from build123d import *

# Parameters (mm, degrees)
F0_W     = 58.42
F0_H     = 31.75
F2_DEPTH = 25.4
F3_R     = 6.35
F4_T     = -3.175
F5_R     = 2.54
F6_DEPTH = 6.35
F7_R     = 1.27
F8_DEPTH = 3.81


with BuildPart() as f2:
    # F0 (on Front) → F2 (new body)
    with BuildSketch(Plane.XZ):
        Rectangle(F0_W, F0_H)
    extrude(amount=F2_DEPTH)

    # F3
    f3_edges = [f2.edges().sort_by_distance(p)[0] for p in [
        (29.21, -12.7, 15.875),
        (29.21, -12.7, -15.875),
        (-29.21, -12.7, 15.875),
        (-29.21, -12.7, -15.875),
    ]]
    fillet(f3_edges, radius=F3_R)

    # F4
    f4_openings = [f2.faces().sort_by_distance(p)[0] for p in [
        (0, -25.4, 0),
    ]]
    offset(amount=F4_T, openings=f4_openings)

    # F5 (on face) → F6 (join)
    with BuildSketch(Plane.XZ.offset(3.175)):
        with Locations((-22.86, 8.89)):
            Circle(F5_R)
        with Locations((22.86, 8.89)):
            Circle(F5_R)
        with Locations((-22.86, -8.89)):
            Circle(F5_R)
        with Locations((22.86, -8.89)):
            Circle(F5_R)
    extrude(amount=F6_DEPTH)

    # F7 (on face) → F8 (join)
    with BuildSketch(Plane.XZ.offset(9.525)):
        with Locations((-22.86, 8.89)):
            Circle(F7_R)
        with Locations((-22.86, -8.89)):
            Circle(F7_R)
        with Locations((22.86, -8.89)):
            Circle(F7_R)
        with Locations((22.86, 8.89)):
            Circle(F7_R)
    extrude(amount=F8_DEPTH)


solid = f2.part
The model under review builds one solid part; all positions refer to its coordinate system, in mm. A direction names the side the tool comes from. Give positions to 0.01 mm unless a question says otherwise; leave off trailing zeros. Write each loop counter-clockwise with the first axis right and the second up, starting at its lowest first coordinate (ties: lowest second). Pieces come first, ordered by that corner, then holes.
1. Draft analysis for pull direction X (two halves, no side actions). For faces 1 (the cylindrical face through (25.13, -14.443, 11.745)), 2 (the cylindrical face through (27.399, -12.878, 13.965)), 3 (the flat face through (0, -13, -15.875)), 4 (the flat face through (-29.21, -13, 0)), state which applies: +X half, -X half, draft (parallel to the pull), parting line (faces both ways), or undercut.
2. For P1, Ø1.3, axis at x = 23, z = 8.5, coming from the -Y side (3 decimals); P2, Ø12.5, axis at x = -8, z = 6, coming from the -Y side (3 decimals), all flat-tipped, find the tip position at first contact; note any pin that passes through.
3. Add section A-A, the plane y = -7.25. Write out the cut boundary in (x, z) (3 decimals), plus the area to 3 significant figures.
4. Add section D-D, the plane x = 17. Write out the cut boundary in (y, z) (3 decimals), plus the area to 3 significant figures.
5. Wall thickness on L1, parallel to Z at x = 10, y = -12.5 (3 decimals); L2, parallel to X at y = -9.5, z = -1 (3 decimals); L3, parallel to X at y = -5, z = 11: over which ranges is each line inside the solid? List them lowest first.
6. Add section B-B, the plane z = -3.5. Write out the cut boundary in (x, y) (3 decimals).
7. Tool access review of faces 5 (the flat face through (23, -13.335, 9)), 6 (the flat face through (0, -13, 15.875)): name each direction out of +Z, -Z, +X, -X, +Y, -Y from which nothing blocks a thin tool from reaching the whole face with its end or side.
8. Add section C-C, the plane y = -17. Write out the cut boundary in (x, z) (3 decimals).
Worked answers:
1. face 1: undercut
1. face 2: +X half
1. face 3: draft
1. face 4: -X half
2. P1: stops at y = -13.335
2. P2: stops at y = -3.175
3. outline: (-29.21, -9.525) arc R6.35 ccw to (-22.86, -15.875) - (22.86, -15.875) arc R6.35 ccw to (29.21, -9.525) - (29.21, 9.525) arc R6.35 ccw to (22.86, 15.875) - (-22.86, 15.875) arc R6.35 ccw to (-29.21, 9.525) - close; circle Ø5.08 at (-22.86, -8.89); circle Ø5.08 at (-22.86, 8.89); circle Ø5.08 at (22.86, -8.89); circle Ø5.08 at (22.86, 8.89); hole (-26.035, -9.525) arc R3.175 ccw to (-22.86, -12.7) - (22.86, -12.7) arc R3.175 ccw to (26.035, -9.525) - (26.035, 9.525) arc R3.175 ccw to (22.86, 12.7) - (-22.86, 12.7) arc R3.175 ccw to (-26.035, 9.525) - close
3. area: 587 mm2
4. outline: (-25.4, -15.875) - (0, -15.875) - (0, 15.875) - (-25.4, 15.875) - (-25.4, 12.7) - (-3.175, 12.7) - (-3.175, -12.7) - (-25.4, -12.7) - close
4. area: 242 mm2
5. L1: z = -15.875 to -12.7, 12.7 to 15.875
5. L2: x = -29.21 to -26.035, 26.035 to 29.21
5. L3: x = -29.04 to -25.67, -24.27 to -21.45, 21.45 to 24.27, 25.67 to 29.04
6. outline: (-29.21, -25.4) - (-26.035, -25.4) - (-26.035, -3.175) - (26.035, -3.175) - (26.035, -25.4) - (29.21, -25.4) - (29.21, 0) - (-29.21, 0) - close
7. face 5: -Y
7. face 6: +Z, +X, -X, +Y, -Y
8. outline: (-29.21, -9.525) arc R6.35 ccw to (-22.86, -15.875) - (22.86, -15.875) arc R6.35 ccw to (29.21, -9.525) - (29.21, 9.525) arc R6.35 ccw to (22.86, 15.875) - (-22.86, 15.875) arc R6.35 ccw to (-29.21, 9.525) - close; hole (-26.035, -9.525) arc R3.175 ccw to (-22.86, -12.7) - (22.86, -12.7) arc R3.175 ccw to (26.035, -9.525) - (26.035, 9.525) arc R3.175 ccw to (22.86, 12.7) - (-22.86, 12.7) arc R3.175 ccw to (-26.035, 9.525) - close
